from build123d import *

# Parameters (mm, degrees)
F0_W     = 195.58
F0_H     = 238.76
F1_DEPTH = 101.6
F3_DEPTH = 195.58


# Not quite as in the source:
# - a pattern or mirror of a feature is missing from the dataset's text; its kind, count and spacing are read off the source's solid


with BuildPart() as f1:
    # F0 (on Top) → F1 (new body)
    with BuildSketch(Plane.XY):
        Rectangle(F0_W, F0_H)
    extrude(amount=F1_DEPTH)

    # F2 (on face) → F3 (join)
    with BuildSketch(Plane(origin=(-97.79, 0, 0), x_dir=(0, -1, 0), z_dir=(-1, 0, 0))):
        Polygon((122.3456934094, 0), (105.8921615149, 0), (105.8921615149, -1.5875), (121.2054859035, -1.5875), (128.7959814072, -7.62), (138.43, -7.62), (138.43, -6.0325), (129.9361889131, -6.0325), align=None)
    f3 = extrude(amount=-F3_DEPTH)

    # F3_copies: F3 across plane
    add(f3.mirror(Plane.ZX))


solid = f1.part
Here's how the part is built. I have some questions about the finished solid (model axes, mm). A direction names the side the tool comes from. Round coordinates to 2 decimals unless told otherwise and drop trailing zeros. Write each loop counter-clockwise with the first axis right and the second up, starting at its lowest first coordinate (ties: lowest second). Pieces come first, ordered by that corner, then holes. Notation, with made-up numbers: (-23, 8) -> (35, 8) arc R30 ccw to (35, 33) -> close; hole circle Ø10 at (16, 32). An arc over 180 degrees is marked (long way). One line per item, written item: value.
1) If I drill on line 1 (Z direction, x = -36.5, y = -12); line 2 (Z direction, x = -30, y = -112); line 3 (Y direction, x = 23, z = 67), over which ranges is the centre line in solid material (lowest first)? Write a range as [from, to].
Filled sheet:
line 1: z = [0, 101.6]
line 2: z = [-1.59, 101.6]
line 3: y = [-119.38, 119.38]
2) For faces 4 (the face through (-1, 134, -7.62)), 5 (the face through (-1.369, 124.948, -4.562)), 6 (the face through (-1, -119.38, 50)), 7 (the face through (-1, 134, -6.032)), which set-ups out of +Z, -Z, +X, -X, +Y, -Y let a thin tool reach every point of the face, with its end or its side?
Filled sheet:
face 4: -Z, +X, -X, +Y, -Y
face 5: -Z, +X, -X
face 6: +Z, +X, -X, -Y
face 7: +Z, +X, -X, +Y
3) Suppose I cut it at A-A on x = -55.5. List the corners of the cut face in (y, z) for me, plus the area to 3 significant figures.
Filled sheet:
outline: (-138.43, -7.62) -> (-128.8, -7.62) -> (-121.21, -1.59) -> (-105.89, -1.59) -> (-105.89, 0) -> (105.89, 0) -> (105.89, -1.59) -> (121.21, -1.59) -> (128.8, -7.62) -> (138.43, -7.62) -> (138.43, -6.03) -> (129.94, -6.03) -> (122.35, 0) -> (119.38, 0) -> (119.38, 101.6) -> (-119.38, 101.6) -> (-119.38, 0) -> (-122.35, 0) -> (-129.94, -6.03) -> (-138.43, -6.03) -> close
area: 24,400 mm2
4) I'm going to push flat-ended pins straight in: pin 1 Ø12.5 at (x, y) = (-47.5, 117) entering from -Z; pin 2 Ø12 at (x, z) = (28.5, 22.5) entering from +Y; pin 3 Ø7 at (x, y) = (12, 133.5) entering from +Z; pin 4 Ø3.5 at (x, y) = (28.5, -121) entering from +Z. Where does each tip first touch, or does it pass through?
Filled sheet:
pin 1: stops at z = -3.21
pin 2: stops at y = 119.38
pin 3: stops at z = -6.03
pin 4: stops at z = 101.6
5) Suppose I cut it at B-B on z = 67. List the corners of the cut face in (x, y) for me, plus the area to 3 significant figures.
Filled sheet:
outline: (-97.79, -119.38) -> (97.79, -119.38) -> (97.79, 119.38) -> (-97.79, 119.38) -> close
area: 46,700 mm2
6) Suppose I cut it at C-C on y = 93.5. List the corners of the cut face in (x, z) for me.
Filled sheet:
outline: (-97.79, 0) -> (97.79, 0) -> (97.79, 101.6) -> (-97.79, 101.6) -> close
7) We'd pull the mould along Y, two halves only. Please class faces 1 (the face through (-1, 119.38, 50)), 2 (the face through (-1, -113, -1.588)), 3 (the face through (-1, -134, -6.032)): released by +Y, released by -Y, zero draft, split by the parting line, or undercut.
Filled sheet:
face 1: released by +Y
face 2: undercut
face 3: zero draft
